Work out the finished part from the listing and answer in its coordinate system (mm). A direction names the side the tool comes from. Round coordinates to 2 decimals unless told otherwise and drop trailing zeros. Loops run counter-clockwise (first coordinate to the right, second up) from the corner with the lowest first, then second, coordinate; pieces in that order, holes last. Notation, with made-up numbers: (-19, 4) -> (8, 4) arc R33 cw to (8, 33) -> close; hole circle Ø9 at (-26, 58). An arc over 180 degrees is marked (long way). Use one line per item in the form item = value.
Autodesk Inventor part; units mm, degrees
ref_plane "工作平面1" through (0, 0, 31) normal (0, 0, 1) x (1, 0, 0)
ref_plane "YZ Plane" through (0, 0, 0) normal (1, 0, 0) x (0, 1, 0)
ref_plane "XZ Plane" through (0, 0, 0) normal (0, 1, 0) x (-1, 0, 0)
sketch "草图1" plane through (0, 0, 0) normal (0, 0, 1) x (1, 0, 0)
  circle A0 centre (0, 0) radius 15.25
  dimension "d0" = 30.5
extrude "拉伸1" add sketch "草图1" along normal blind 62
sketch "草图2" plane through (0, 0, 62) normal (0, 0, 1) x (1, 0, 0)
  arc A0 (5.1473, -3.0831) -> (5.1473, 3.0831) centre (0, 0) ccw
  arc A1 (10.7235, -6.423) -> (10.7235, 6.423) centre (0, 0) ccw
  line L0 (5.1473, 3.0831) -> (10.7235, 6.423)
  line L1 (0, 0) -> (24.4496, 0) construction
  line L2 (5.1473, -3.0831) -> (10.7235, -6.423)
  line L3 (-5.2437, 2.9162) -> (-10.9243, 6.0753)
  arc A2 (0.0964, 5.9992) -> (-5.2437, 2.9162) centre (0, 0) ccw
  line L4 (0.0964, 5.9992) -> (0.2008, 12.4984)
  arc A3 (0.2008, 12.4984) -> (-10.9243, 6.0753) centre (0, 0) ccw
  line L5 (0.0964, -5.9992) -> (0.2008, -12.4984)
  arc A4 (-5.2437, -2.9162) -> (0.0964, -5.9992) centre (0, 0) ccw
  line L6 (-5.2437, -2.9162) -> (-10.9243, -6.0753)
  arc A5 (-10.9243, -6.0753) -> (0.2008, -12.4984) centre (0, 0) ccw
  dimension "d4" = 12
  dimension "d5" = 30.92
  dimension "d8" = 360
  dimension "d16" = 12.5
extrude "拉伸2" cut sketch "草图2" against normal through all
sketch "草图3" plane through (0, 0, 62) normal (0, 0, 1) x (1, 0, 0)
  arc A0 (1, 1.249) -> (1, -1.249) centre (0, 0) ccw
  line L0 (1, 1.249) -> (1, -1.249)
  line L1 (-1.6, 0) -> (-1.6, 2.5625) construction
  dimension "d12" = 3.2
  dimension "d13" = 2.6
extrude "拉伸3" cut sketch "草图3" against normal blind 9.2
ref_plane "工作平面1" through (0, 0, 31) normal (0, 0, 1) x (1, 0, 0)
mirror "镜像1" about plane through (0, 0, 31) normal (0, 0, 1) of "拉伸3"
properties part number "滚轮内轮" material "尼龙 6/6"
(1) Find section D-D, the plane x = -10. Write down the section's boundary in (y, z), then the cut area to 3 significant figures.
Completed:
outline = (-11.51, 0) -> (-7.5, 0) -> (-7.5, 62) -> (-11.51, 62) -> close; (-5.56, 0) -> (5.56, 0) -> (5.56, 62) -> (-5.56, 62) -> close; (7.5, 0) -> (11.51, 0) -> (11.51, 62) -> (7.5, 62) -> close
area = 1,190 mm2
(2) Consider L1, parallel to Y at x = 0, z = 3; L2, parallel to X at y = 3, z = 14; L3, parallel to Y at x = -8, z = 30. Determine where each line is inside the solid, lowest interval first.
Completed:
L1 = -15.25 to -12.5, -6 to -1.6, 1.6 to 6, 12.5 to 15.25
L2 = -14.95 to -5.39, -5.2 to 5.2, 12.13 to 14.95
L3 = -12.98 to -9.6, -4.45 to 4.45, 9.6 to 12.98
(3) Find section C-C, the plane x = 8. Write down the section's boundary in (y, z).
Completed:
outline = (-12.98, 0) -> (-4.79, 0) -> (-4.79, 62) -> (-12.98, 62) -> close; (4.79, 0) -> (12.98, 0) -> (12.98, 62) -> (4.79, 62) -> close
(4) For a pull along Y with two mould halves and no side action, classify faces 4 (the cylindrical face through (-12.1, 9.28, 30.57)), 5 (the flat face through (7.9, -4.73, 31.43)), 6 (the cylindrical face through (-2.96, 5.22, 31.43)), 7 (the flat face through (3, 0, 0)) as +Y half, -Y half, draft (parallel to the pull), parting line (faces both ways), or undercut.
Completed:
face_4 = parting line
face_5 = undercut
face_6 = undercut
face_7 = draft
(5) Find section A-A, the plane z = 33.5. Write down the section's boundary in (x, y), then the cut area to 3 significant figures.
Completed:
outline = circle Ø30.5 at (0, 0); hole (-10.92, -6.08) arc R12.5 ccw to (0.2, -12.5) -> (0.1, -6) arc R6 cw to (-5.24, -2.92) -> close; hole (-10.92, 6.08) -> (-5.24, 2.92) arc R6 cw to (0.1, 6) -> (0.2, 12.5) arc R12.5 ccw to start; hole (5.15, -3.08) -> (10.72, -6.42) arc R12.5 ccw to (10.72, 6.42) -> (5.15, 3.08) arc R6 cw to start
area = 536 mm2
(6) For faces 1 (the flat face through (0, 0, 9.2)), 2 (the flat face through (0, 0, 52.8)), 3 (the cylindrical face through (-6.33, -10.78, 31.43)), determine the directions among +Z, -Z, +X, -X, +Y, -Y from which every point of the face is accessible in a straight line to the end or side of a thin tool.
Completed:
face_1 = -Z
face_2 = +Z
face_3 = +Z, -Z
(7) Find section B-B, the plane y = 0. Write down the section's boundary in (x, z).
Completed:
outline = (-15.25, 0) -> (-1.6, 0) -> (-1.6, 9.2) -> (1, 9.2) -> (1, 0) -> (6, 0) -> (6, 62) -> (1, 62) -> (1, 52.8) -> (-1.6, 52.8) -> (-1.6, 62) -> (-15.25, 62) -> close; (12.5, 0) -> (15.25, 0) -> (15.25, 62) -> (12.5, 62) -> close
(8) Given P1, Ø4, axis at y = -6, z = 32.5, coming from the -X side; P2, Ø0.8, axis at x = -0.5, y = -0.5, coming from the +Z side; P3, Ø0.8, axis at x = 0, y = 0.5, coming from the -Z side, each flat-ended and moving along its own axis, determine where each tip first touches the part or whether it passes through.
Completed:
P1 = -14.72
P2 = 52.8
P3 = 9.2
